```python
from build123d import *

# Parameters (mm, degrees)
F1_DEPTH = 6.35
F2_R     = 9.525
F3_DEPTH = 6.351
F5_DEPTH = 6.351


with BuildPart() as f1:
    # F0 (on Top) → F1 (new body)
    with BuildSketch(Plane.XY):
        with BuildLine():
            ThreePointArc((76.2, 44.45), (72.480256, 53.430256), (63.5, 57.15))
            Line((63.5, 57.15), (-63.5, 57.15))
            ThreePointArc((-63.5, 57.15), (-72.480256, 53.430256), (-76.2, 44.45))
            Line((-76.2, 44.45), (-76.2, -44.45))
            ThreePointArc((-76.2, -44.45), (-72.480256, -53.430256), (-63.5, -57.15))
            Line((-63.5, -57.15), (63.5, -57.15))
            ThreePointArc((63.5, -57.15), (72.480256, -53.430256), (76.2, -44.45))
            Line((76.2, -44.45), (76.2, 44.45))
        make_face()
    extrude(amount=F1_DEPTH)

    # F2 (on face) → F3 (cut, through all)
    with BuildSketch(Plane.XY.offset(6.35)):
        with Locations((38.1, 31.75)):
            Circle(F2_R)
        with Locations((38.1, 0)):
            Circle(F2_R)
        with Locations((38.1, -31.75)):
            Circle(F2_R)
    extrude(amount=-F3_DEPTH, mode=Mode.SUBTRACT)

    # F4 (on face) → F5 (cut, through all)
    with BuildSketch(Plane.XY.offset(6.35)):
        with BuildLine():
            Line((-59.763934, -48.186066), (-9.324066, -48.186066))
            ThreePointArc((-9.324066, -48.186066), (-5.588, -44.45), (-9.324066, -40.713934))
            Line((-9.324066, -40.713934), (-59.763934, -40.713934))
            ThreePointArc((-59.763934, -40.713934), (-63.5, -44.45), (-59.763934, -48.186066))
        make_face()
        with BuildLine():
            ThreePointArc((-59.763934, -28.013934), (-63.5, -31.75), (-59.763934, -35.486066))
            Line((-59.763934, -35.486066), (-9.324066, -35.486066))
            ThreePointArc((-9.324066, -35.486066), (-5.588, -31.75), (-9.324066, -28.013934))
            Line((-9.324066, -28.013934), (-59.763934, -28.013934))
        make_face()
        with BuildLine():
            ThreePointArc((-59.763934, -15.313934), (-63.5, -19.05), (-59.763934, -22.786066))
            Line((-59.763934, -22.786066), (-9.324066, -22.786066))
            ThreePointArc((-9.324066, -22.786066), (-5.588, -19.05), (-9.324066, -15.313934))
            Line((-9.324066, -15.313934), (-59.763934, -15.313934))
        make_face()
        with BuildLine():
            ThreePointArc((-59.763934, -2.613934), (-63.5, -6.35), (-59.763934, -10.086066))
            Line((-59.763934, -10.086066), (-9.324066, -10.086066))
            ThreePointArc((-9.324066, -10.086066), (-5.588, -6.35), (-9.324066, -2.613934))
            Line((-9.324066, -2.613934), (-59.763934, -2.613934))
        make_face()
        with BuildLine():
            ThreePointArc((-59.763934, 10.086066), (-63.5, 6.35), (-59.763934, 2.613934))
            Line((-59.763934, 2.613934), (-9.324066, 2.613934))
            ThreePointArc((-9.324066, 2.613934), (-5.588, 6.35), (-9.324066, 10.086066))
            Line((-9.324066, 10.086066), (-59.763934, 10.086066))
        make_face()
        with BuildLine():
            ThreePointArc((-59.763934, 22.786066), (-63.5, 19.05), (-59.763934, 15.313934))
            Line((-59.763934, 15.313934), (-9.324066, 15.313934))
            ThreePointArc((-9.324066, 15.313934), (-5.588, 19.05), (-9.324066, 22.786066))
            Line((-9.324066, 22.786066), (-59.763934, 22.786066))
        make_face()
        with BuildLine():
            ThreePointArc((-59.763934, 35.486066), (-63.5, 31.75), (-59.763934, 28.013934))
            Line((-59.763934, 28.013934), (-9.324066, 28.013934))
            ThreePointArc((-9.324066, 28.013934), (-5.588, 31.75), (-9.324066, 35.486066))
            Line((-9.324066, 35.486066), (-59.763934, 35.486066))
        make_face()
        with BuildLine():
            ThreePointArc((-59.763934, 48.186066), (-63.5, 44.45), (-59.763934, 40.713934))
            Line((-59.763934, 40.713934), (-9.324066, 40.713934))
            ThreePointArc((-9.324066, 40.713934), (-5.588, 44.45), (-9.324066, 48.186066))
            Line((-9.324066, 48.186066), (-59.763934, 48.186066))
        make_face()
    extrude(amount=-F5_DEPTH, mode=Mode.SUBTRACT)


solid = f1.part
```
Geometry check sheet. Reference: the model listing, model coordinates, mm. A direction names the side the tool comes from. Coordinates: 2 decimals unless noted, no trailing zeros. Write each loop counter-clockwise with the first axis right and the second up, starting at its lowest first coordinate (ties: lowest second). Pieces come first, ordered by that corner, then holes. Notation, with made-up numbers: (13.25, -35.5) -> (68.25, -35.5) arc R15 cw to (68.25, -8.5) -> close; hole circle Ø4 at (8.5, 6). An arc over 180 degrees is marked (long way). Use CSV: the item, a comma, the result in double quotes. Start each with the question number.
Item 1: Cross-section at C-C, the plane z = 5. State how many separate pieces and enclosed holes the cut face has, plus the area to 3 significant figures.
Item 2: Thickness scan on line 1 (Y direction, x = 38.1, z = 4.5) (3 decimals); line 2 (X direction, y = 5, z = 2.25); line 3 (X direction, y = -23.5, z = 2.75). Record the ranges inside material, lowest first.
Item 3: Mould release check, pull along Y, two halves, no side actions. Record for faces 3 (the flat face through (-34, -2.614, 3)), 4 (the flat face through (76.2, -1, 3)), 5 (the cylindrical face through (-72.38, 53.53, 3.13)): released by +Y, released by -Y, zero draft, split by the parting line, or undercut.
Item 4: Cross-section at A-A, the plane y = 19.05. Record the cut outline in (x, z), plus the area to 3 significant figures.
Item 5: Cross-section at B-B, the plane y = 31.75. Record the cut outline in (x, z) (3 decimals), plus the area to 3 significant figures.
Item 6: Set-up check for faces 1 (the cylindrical face through (-72.58, -53.33, 3.13)), 2 (the flat face through (-34, 35.486, 3)): record each of +Z, -Z, +X, -X, +Y, -Y from which the full face is reachable in a straight line by a thin tool's end or side.
Item 7: Depth check by flat-ended pin: pin 1 Ø3 at (x, y) = (57.5, 44) entering from -Z; pin 2 Ø15 at (x, y) = (38.1, -31.75) entering from -Z. Enter the tip coordinate at first touch or a pass-through.
Answers:
1,separate pieces,"1"
1,enclosed holes,"11"
1,area,"13,100 mm^2"
2,line 1,"-57.15 to -41.275, -22.225 to -9.525, 9.525 to 22.225, 41.275 to 57.15"
2,line 2,"-76.2 to -63.25, -5.84 to 29.99, 46.21 to 76.2"
2,line 3,"-76.2 to 33.34, 42.86 to 76.2"
3,face 3,"undercut"
3,face 4,"zero draft"
3,face 5,"released by +Y"
4,outline,"(-76.2, 0) -> (-63.5, 0) -> (-63.5, 6.35) -> (-76.2, 6.35) -> close; (-5.59, 0) -> (76.2, 0) -> (76.2, 6.35) -> (-5.59, 6.35) -> close"
4,area,"600 mm^2"
5,outline,"(-76.2, 0) -> (-63.5, 0) -> (-63.5, 6.35) -> (-76.2, 6.35) -> close; (-5.588, 0) -> (28.575, 0) -> (28.575, 6.35) -> (-5.588, 6.35) -> close; (47.625, 0) -> (76.2, 0) -> (76.2, 6.35) -> (47.625, 6.35) -> close"
5,area,"479 mm^2"
6,face 1,"+Z, -Z, -X, -Y"
6,face 2,"+Z, -Z"
7,pin 1,"z = 0"
7,pin 2,"through"
